Check sheet for the modelled part. Datum: model origin and axes. Units: mm. A direction names the side the tool comes from. Give positions to 0.01 mm unless a question says otherwise; leave off trailing zeros. Order: outer loops, then holes, each group sorted by start corner. A loop starts at its lowest first (then second) coordinate and runs counter-clockwise, first axis right, second up.
Item 1: Sectioned sample at C-C on x = 18. Record the boundary of the cut face in (y, z).
Item 2: Sectioned sample at B-B on x = 2.75. Record the boundary of the cut face in (y, z).
Item 3: Gauge pin test, flat ends, axial feed: P1, Ø3, axis at x = 3.5, y = 1, coming from the +Z side; P2, Ø3, axis at x = 18, z = 0, coming from the +Y side; P3, Ø3, axis at x = 13.5, y = 2.5, coming from the +Z side. Record the tip position at first contact, or that the pin passes through.
Item 4: Access from +Z, -Z, +X, -X, +Y, -Y to the whole of each face (thin tool, end or side, straight path). Record for faces 5 (the cylindrical face through (16, -1, 0)), 6 (the cylindrical face through (-1.51, -1.08, 4.88)), 7 (the cylindrical face through (-4, -3, 0)).
Item 5: Release check for a two-part mould opening along X. For faces 1 (the cylindrical face through (18.05, 1.45, 1.25)), 2 (the cylindrical face through (1.49, -1.08, 4.88)), 3 (the cylindrical face through (-0.01, -0.59, -4.46)), 4 (the flat face through (21, 0, 1.2)) record: released by +X, released by -X, zero draft, split by the parting line, or undercut.
Item 6: Sectioned sample at A-A on x = 14.25. Record the boundary of the cut face in (y, z).
Item 7: Material ranges on line 1 along X through (y, z) = (1.85, 0); line 2 along Z through (x, y) = (15.75, 0); line 3 along X through (y, z) = (0, -4.25), recorded low to high.
from build123d import *

# Parameters (mm, degrees)
FASE1_SIZE               = 0.5
M3_GEWINDEBOHRUNG1_D     = 2.5
M3_GEWINDEBOHRUNG1_DEPTH = 3
M3_GEWINDEBOHRUNG1_TIP   = 0.751075774
FASE2_SIZE               = 0.2


with BuildPart() as part:
    # Skizze1 → Rotation1 (revolve)
    with BuildSketch(Plane.XY):
        Polygon((-3, 3), (-6, 3), (-6, 0), (11, 0), (11, 1), (21, 1), (21, 2.95), (6, 2.95), (6, 3), (3, 3), (3, 3.5), (2.5, 3.5), (2.5, 5), (1, 5), (0.5, 4.5), (-0.5, 4.5), (-1, 5), (-2.5, 5), (-2.5, 3.5), (-3, 3.5), align=None)
    revolve(axis=Axis((-5.518776228, 0, 0), (-1, 0, 0)))

    # Fase1
    fase1_edges = [part.edges().sort_by_distance(p)[0] for p in [
        (2.5, -5, 0),
        (-2.5, -5, 0),
    ]]
    chamfer(fase1_edges, length=FASE1_SIZE)

    # M3 Gewindebohrung1
    with Locations(Plane(origin=(18, 3, 0), x_dir=(0, 0, 1), z_dir=(0, 1, 0))):
        with Locations((0, 0)):
            Hole(M3_GEWINDEBOHRUNG1_D / 2, depth=M3_GEWINDEBOHRUNG1_DEPTH)
            with Locations((0, 0, -(M3_GEWINDEBOHRUNG1_DEPTH + M3_GEWINDEBOHRUNG1_TIP / 2))):  # 118° drill point
                Cone(0, M3_GEWINDEBOHRUNG1_D / 2, M3_GEWINDEBOHRUNG1_TIP, mode=Mode.SUBTRACT)

    # Fase2
    fase2_edges = [part.edges().sort_by_distance(p)[0] for p in [
        (-6, -3, 0),
        (21, -2.95, 0),
    ]]
    chamfer(fase2_edges, length=FASE2_SIZE)


solid = part.part
Report:
1. outline: (-0.16, -0.99) arc R1 cw to (-0.16, 0.99) - (0, 1.25) - (2.67, 1.25) arc R2.95 ccw (long way) to (2.67, -1.25) - (0, -1.25) - close
2. outline: circle Ø7 at (0, 0)
3. P1: stops at z = 4.92
3. P2: stops at y = 2.95
3. P3: stops at z = 2.78
4. face 5: +X
4. face 6: +X, -X
4. face 7: -X
5. face 1: undercut
5. face 2: zero draft
5. face 3: undercut
5. face 4: released by +X
6. outline: circle Ø5.9 at (0, 0); hole circle Ø2 at (0, 0)
7. line 1: x = -6 to 16.75, 19.25 to 21
7. line 2: z = -2.95 to -1, 1 to 2.95
7. line 3: x = -2.5 to 2.5
